from build123d import *

# Parameters (mm, degrees)
SKETCH1_R           = 4.7625
BOSS_EXTRUDE1_DEPTH = 4.7625
SKETCH1_2_R         = 4.7625
SKETCH1_2_R_2       = 3.3734375
BOSS_EXTRUDE2_DEPTH = 2.032


with BuildPart() as part:
    # Sketch1 → Boss-Extrude1 (new body)
    with BuildSketch(Plane.XY):
        with BuildLine():
            Line((-73.66, 7.9375), (73.66, 7.9375))
            ThreePointArc((73.66, 7.9375), (81.5975, 0), (73.66, -7.9375))
            Line((73.66, -7.9375), (-73.66, -7.9375))
            ThreePointArc((-73.66, -7.9375), (-81.5975, 0), (-73.66, 7.9375))
        make_face()
        with Locations(Location((73.66, 0, 0), (0, 0, 180))):
            Circle(SKETCH1_R, mode=Mode.SUBTRACT)
        with Locations(Location((-73.66, 0, 0), (0, 0, 180))):
            Circle(SKETCH1_R, mode=Mode.SUBTRACT)
        with Locations(Location((0, 0, 0), (0, 0, 180))):
            Circle(SKETCH1_R, mode=Mode.SUBTRACT)
    extrude(amount=BOSS_EXTRUDE1_DEPTH)

    # Sketch1_2 → Boss-Extrude2 (add)
    with BuildSketch(Plane.XY):
        with Locations(Location((-73.66, 0, 0), (0, 0, 180))):
            Circle(SKETCH1_2_R)
        with Locations((-73.66, 0)):
            Circle(SKETCH1_2_R_2, mode=Mode.SUBTRACT)
    extrude(amount=BOSS_EXTRUDE2_DEPTH)


solid = part.part
Geometry: final body of the model. Coordinates: model frame, mm. A direction names the side the tool comes from. Give positions to 0.01 mm unless a question says otherwise; leave off trailing zeros. Loops run counter-clockwise (first coordinate to the right, second up) from the corner with the lowest first, then second, coordinate; pieces in that order, holes last. Notation, with made-up numbers: (-27.5, 8) - (24.5, 8) arc R8 cw to (24.5, 21) - close; hole circle Ø7 at (-15, -22.75). An arc over 180 degrees is marked (long way). Answer as CSV lines item,"result". Start each with the question number.
1. Ray query, L1, parallel to X at y = -1.25, z = 2.2; L2, parallel to X at y = 2.75, z = 3.35; L3, parallel to Y at x = -73.66, z = 0.5. Return the intervals inside material, ascending.
2. Section C-C, the plane y = -1.5. Return loops of the section in (x, z), plus the area to 3 significant figures.
3. Section B-B, the plane x = 0. Return loops of the section in (y, z).
4. Section A-A, the plane z = 1. Return loops of the section in (x, y) (1 decimal), plus the area to 3 significant figures.
5. Pin query (flat end, axial travel): P1, Ø1.5, axis at x = -0.5, y = -5.5, coming from the -Z side; P2, Ø7.5, axis at x = -73.66, y = 0, coming from the +Z side. Return the tip coordinate at first contact, or that it passes through.
6. Reachability of faces 4 (the face through (1, 5, 4.762)), 5 (the face through (-70, 1, 2.032)) from +Z, -Z, +X, -X, +Y, -Y: full face, straight path, thin tool, end or side. Return the list, or none.
7. Draft query along X for faces 1 (the face through (-81.596, -0.175, 2.348)), 2 (the face through (-1, 7.938, 2)), 3 (the face through (-77.03, 0.15, 1)). Return one class per face: released by +X, released by -X, zero draft, split by the parting line, or undercut.
Answers:
1,L1,"x = -81.5 to -78.26, -69.06 to -4.6, 4.6 to 69.06, 78.26 to 81.5"
1,L2,"x = -81.11 to -77.55, -69.77 to -3.89, 3.89 to 69.77, 77.55 to 81.11"
1,L3,"y = -7.94 to -3.37, 3.37 to 7.94"
2,outline,"(-81.45, 0) - (-76.68, 0) - (-76.68, 2.03) - (-78.18, 2.03) - (-78.18, 4.76) - (-81.45, 4.76) - close; (-70.64, 0) - (-4.52, 0) - (-4.52, 4.76) - (-69.14, 4.76) - (-69.14, 2.03) - (-70.64, 2.03) - close; (4.52, 0) - (69.14, 0) - (69.14, 4.76) - (4.52, 4.76) - close; (78.18, 0) - (81.45, 0) - (81.45, 4.76) - (78.18, 4.76) - close"
2,area,"653 mm2"
3,outline,"(-7.94, 0) - (-4.76, 0) - (-4.76, 4.76) - (-7.94, 4.76) - close; (4.76, 0) - (7.94, 0) - (7.94, 4.76) - (4.76, 4.76) - close"
4,outline,"(-73.7, -7.9) - (73.7, -7.9) arc R7.9 ccw to (73.7, 7.9) - (-73.7, 7.9) arc R7.9 ccw to start; hole circle Ø6.7 at (-73.7, 0); hole circle Ø9.5 at (0, 0); hole circle Ø9.5 at (73.7, 0)"
4,area,"2,360 mm2"
5,P1,"stops at z = 0"
5,P2,"stops at z = 2.03"
6,face 4,"+Z, +X, -X, +Y, -Y"
6,face 5,"+Z"
7,face 1,"released by -X"
7,face 2,"zero draft"
7,face 3,"undercut"
